from build123d import *

# Parameters (mm, degrees)
SKETCH1_R           = 3.2385
BOSS_EXTRUDE1_DEPTH = 6.35
CUT_EXTRUDE1_DEPTH  = 2.2


with BuildPart() as part:
    # Sketch1 → Boss-Extrude1 (new body)
    with BuildSketch(Plane.XY):
        with BuildLine():
            Line((7.9756, 23.114), (7.9756, -23.114))
            ThreePointArc((7.9756, -23.114), (0, -31.0896), (-7.9756, -23.114))
            Line((-7.9756, -23.114), (-7.9756, 23.114))
            ThreePointArc((-7.9756, 23.114), (0, 31.0896), (7.9756, 23.114))
        make_face()
        with Locations((0, 23.114)):
            Circle(SKETCH1_R, mode=Mode.SUBTRACT)
        with Locations((0, -23.114)):
            Circle(SKETCH1_R, mode=Mode.SUBTRACT)
    extrude(amount=BOSS_EXTRUDE1_DEPTH)

    # Sketch2 → Cut-Extrude1 (cut)
    with BuildSketch(Plane.XY.offset(6.35)):
        Polygon((-7.534421013, 23.114), (-3.767210506, 16.589), (3.767210506, 16.589), (7.534421013, 23.114), (3.767210506, 29.639), (-3.767210506, 29.639), align=None)
    extrude(amount=-CUT_EXTRUDE1_DEPTH, mode=Mode.SUBTRACT)


solid = part.part
The model under review builds one solid part; all positions refer to its coordinate system, in mm. A direction names the side the tool comes from. Coordinates: 2 decimals unless noted, no trailing zeros. Loops run counter-clockwise (first coordinate to the right, second up) from the corner with the lowest first, then second, coordinate; pieces in that order, holes last. Notation, with made-up numbers: M -8,-17.75 L 13,-17.75 A31 ccw 13,12.25 Z; hole C 50,35 d3. An arc over 180 degrees is marked long. Put each result on its own line as item: value. Start each with the question number.
Q1. Add section D-D (x = -4.5). Write out the cut boundary in (y, z).
Q2. For faces 1 (the flat face through (7.976, 0, 3)), 2 (the flat face through (5.677, 26.331, 5.265)), list the 3-axis set-ups (+Z, -Z, +X, -X, +Y, -Y) from which the entire face can be reached by the end or side of a thin tool; tool diameter is ignored.
Q3. Clearance check with flat-ended pins moving along their axes: pin 1 (1.5 mm diameter, centred on x = 3, z = 2, fed in from +Y); pin 2 (4 mm diameter, centred on x = 1, y = 24, fed in from +Z); pin 3 (2 mm diameter, centred on x = 3.5, z = 5.5, fed in from -Y). State where each tip first meets the part, or that it passes through.
Q4. Add section A-A (x = 0). Write out the cut boundary in (y, z), and give its area (3 significant figures).
Q5. Add section C-C (x = 2.5). Write out the cut boundary in (y, z), and give its area (3 significant figures).
Q6. The part is to be moulded in two halves that separate along Y. For faces 3 (the cylindrical face through (-0.4, -19.9, 3.1)), 4 (the cylindrical face through (-0.175, 31.088, 3.131)), 5 (the cylindrical face through (0.175, -31.088, 3.131)), 6 (the flat face through (0, -6, 6.35)), say which applies: +Y half, -Y half, draft (parallel to the pull), parting line (faces both ways), or undercut.
Q7. Wall thickness on line 1 (Y direction, x = 0, z = 2.5); line 2 (Y direction, x = 0.25, z = 2.75); line 3 (X direction, y = 20, z = 5): over which ranges is each line inside the solid? List them lowest first.
Q8. Add section B-B (z = 3.25). Write out the cut boundary in (x, y), and give its area (3 significant figures).
Answers:
1. outline: M -29.7,0 L 29.7,0 L 29.7,6.35 L 28.37,6.35 L 28.37,4.15 L 17.86,4.15 L 17.86,6.35 L -29.7,6.35 Z
2. face 1: +Z, -Z, +X, +Y, -Y
2. face 2: +Z
3. pin 1: stops at y = 30.77
3. pin 2: stops at z = 4.15
3. pin 3: stops at y = -30.69
4. outline: M -31.09,0 L -26.35,0 L -26.35,6.35 L -31.09,6.35 Z; M -19.88,0 L 19.88,0 L 19.88,4.15 L 16.59,4.15 L 16.59,6.35 L -19.88,6.35 Z; M 26.35,0 L 31.09,0 L 31.09,6.35 L 29.64,6.35 L 29.64,4.15 L 26.35,4.15 Z
4. area: 298 mm^2
5. outline: M -30.69,0 L -25.17,0 L -25.17,6.35 L -30.69,6.35 Z; M -21.06,0 L 21.06,0 L 21.06,4.15 L 16.59,4.15 L 16.59,6.35 L -21.06,6.35 Z; M 25.17,0 L 30.69,0 L 30.69,6.35 L 29.64,6.35 L 29.64,4.15 L 25.17,4.15 Z
5. area: 318 mm^2
6. face 3: undercut
6. face 4: +Y half
6. face 5: -Y half
6. face 6: draft
7. line 1: y = -31.09 to -26.35, -19.88 to 19.88, 26.35 to 31.09
7. line 2: y = -31.09 to -26.34, -19.89 to 19.89, 26.34 to 31.09
7. line 3: x = -7.98 to -5.74, 5.74 to 7.98
8. outline: M -7.98,-23.11 A7.98 ccw 7.98,-23.11 L 7.98,23.11 A7.98 ccw -7.98,23.11 Z; hole C 0,-23.11 d6.48; hole C 0,23.11 d6.48
8. area: 871 mm^2
